Model file for the job. Use its own axes, mm. A direction names the side the tool comes from. Give positions to 0.01 mm unless a question says otherwise; leave off trailing zeros. Write each loop counter-clockwise with the first axis right and the second up, starting at its lowest first coordinate (ties: lowest second). Pieces come first, ordered by that corner, then holes.
```python
from build123d import *

# Parameters (mm, degrees)
BOSS_EXTRUDE1_DEPTH  = 82.956052622
CHAMFER1_SIZE        = 83.058
CHAMFER1_SIZE_2      = 29.329393675
BOSS_EXTRUDE3_START  = 2.592376644
BOSS_EXTRUDE3_DEPTH  = 72.586546044
CHAMFER6_SIZE        = 72.644
CHAMFER6_SIZE_2      = 25.663219438
BOSS_EXTRUDE19_DEPTH = 25.4
BOSS_EXTRUDE20_DEPTH = 25.4
BOSS_EXTRUDE21_DEPTH = 25.4
BOSS_EXTRUDE23_DEPTH = 25.4
BOSS_EXTRUDE26_START = 38.1
BOSS_EXTRUDE26_DEPTH = 12.7
BOSS_EXTRUDE27_START = -25.4
BOSS_EXTRUDE27_DEPTH = 12.7
MIRROR2_START        = 38.1
MIRROR2_COPY_2_DEPTH = 12.7
MIRROR2_START_2      = -25.4
MIRROR2_COPY_3_DEPTH = 12.7
MIRROR2_COPY_5_DEPTH = 12.7
MIRROR2_COPY_6_DEPTH = 12.7


with BuildPart() as part:
    # Sketch1 → Boss-Extrude1 (new body)
    with BuildSketch(Plane(origin=(0, 0, 0), x_dir=(1, 0, 0), z_dir=(0, 1, 0))):
        Polygon((-50.8, -29.329393675), (0, 58.65878735), (50.8, -29.329393675), align=None)
    extrude(amount=BOSS_EXTRUDE1_DEPTH)

    # Chamfer1
    # the kernel refuses this chamfer: 83.058, 29.329393675 mm, written as the material it takes off along each edge
    with BuildSketch(Plane(origin=(-158.547298904, 82.956052622, 215.953189756), x_dir=(-0.011114252752895883, -0.9999176455327007, -0.006416816818725978), z_dir=(0.5000000000000001, 0, -0.8660254037844387)), Plane(origin=(266.294597809, 82.956052622, 29.329393675), x_dir=(0, -0.9999176455327007, 0.012833633637452178), z_dir=(-1, 0, 0)), Plane(origin=(-107.747298904, 82.956052622, -245.28258343), x_dir=(0.011114252752896008, -0.9999176455327007, -0.006416816818726048), z_dir=(0.49999999999999994, 0, 0.8660254037844387))) as chamfer1_piece_1:
        Polygon((CHAMFER1_SIZE * 0.999917645533, -CHAMFER1_SIZE * 0.0128336336375), (-CHAMFER1_SIZE_2 * 0.0128336336374, -CHAMFER1_SIZE_2 * 0.999917645527), (0, 0), align=None)
    extrude(amount=532.589195618, mode=Mode.SUBTRACT)


with BuildPart() as body_2:
    # Sketch2 → Boss-Extrude3 (new body)
    with BuildSketch(Plane(origin=(0, 0, 0), x_dir=(1, 0, 0), z_dir=(0, 1, 0)).offset(BOSS_EXTRUDE3_START)):
        Polygon((-44.45, -25.663219465), (0, 51.326438931), (44.45, -25.663219465), align=None)
    extrude(amount=BOSS_EXTRUDE3_DEPTH)

    # Chamfer6
    # the kernel refuses this chamfer: 72.644, 25.663219438 mm, written as the material it takes off along each edge
    with BuildSketch(Plane(origin=(-94.237538797, 75.178922689, -214.550644108), x_dir=(0.011118590367512081, -0.9999175812357334, -0.0064193211416922824), z_dir=(0.5000000000000001, 0, 0.8660254037844386)), Plane(origin=(-138.687538797, 75.178922689, 188.887424643), x_dir=(-0.011118590367511921, -0.9999175812357334, -0.006419321141692186), z_dir=(0.49999999999999994, 0, -0.8660254037844387)), Plane(origin=(232.925077595, 75.178922689, 25.663219465), x_dir=(0, -0.9999175812357332, 0.012838642283384548), z_dir=(-1, 0, 0))) as chamfer6_piece_1:
        Polygon((CHAMFER6_SIZE * 0.999917581236, -CHAMFER6_SIZE * 0.0128386422834), (-CHAMFER6_SIZE_2 * 0.0128386422834, -CHAMFER6_SIZE_2 * 0.999917581236), (0, 0), align=None)
    extrude(amount=465.850155189, mode=Mode.SUBTRACT)

    # Sketch19 → Boss-Extrude19 (add)
    with BuildSketch(Plane(origin=(0, 8.341471254, 23.611918188), x_dir=(1, 0, 0), z_dir=(0, 0.3330989621400992, 0.9428918715426434))):
        Polygon((0, 70.885595133), (-44.414844608, -6.097300002), (44.414844608, -6.097300002), align=None)
    extrude(amount=BOSS_EXTRUDE19_DEPTH)

    # Sketch20 → Boss-Extrude20 (add)
    with BuildSketch(Plane(origin=(-20.448520983, 8.341471254, -11.805959094), x_dir=(-0.43652342739361594, 0.1780689969978707, 0.8818949651997697), z_dir=(-0.8165683137777828, 0.3330989621400992, -0.47144593577132166))):
        Polygon((13.387035379, 69.610019986), (42.464106341, -14.375505607), (-44.767106565, 2.400345516), align=None)
    extrude(amount=BOSS_EXTRUDE20_DEPTH)

    # Sketch21 → Boss-Extrude21 (add)
    with BuildSketch(Plane(origin=(20.448520983, 8.341471254, -11.805959094), x_dir=(-0.43652342739361605, -0.1780689969978708, -0.8818949651997696), z_dir=(0.8165683137777828, 0.3330989621400991, -0.47144593577132177))):
        Polygon((-13.387035361, 69.610020002), (-42.464106341, -14.375505607), (44.767106565, 2.400345516), align=None)
    extrude(amount=BOSS_EXTRUDE21_DEPTH)

    # Sketch22 → Boss-Extrude23 (add)
    with BuildSketch(Plane.XZ.offset(-2.592376644)):
        Polygon((44.414844608, 25.64292249), (-44.414844608, 25.64292249), (0, -51.285844981), align=None)
    extrude(amount=BOSS_EXTRUDE23_DEPTH)


with BuildPart() as part_1:
    add(part.part)

    # Combine3: cut body 2
    add(body_2.part, mode=Mode.SUBTRACT)

    # Sweep2: sweep along a path in Sketch25
    with BuildLine(Plane(origin=(0, 0, 0), x_dir=(0, 0, -1), z_dir=(1, 0, 0))) as sweep2_path:
        Line((-29.293394075, 0), (-41.26870121, 4.228713638))
        ThreePointArc((-41.26870121, 4.228713638), (-44.883330876, 7.477532809), (-45.141997958, 12.330724024))
    # Sketch24 → Sweep2 (sweep)
    with BuildSketch(Plane(origin=(0, 9.197233007, 26.045672391), x_dir=(1, 0, 0), z_dir=(0, 0.33296957778049097, 0.9429375696580775))):
        Polygon((-50.737646864, -9.753809057), (50.737646864, -9.753809057), (50.03399067, -8.533709325), (-50.03399067, -8.533709325), align=None)
    sweep2 = sweep(path=sweep2_path.line)

    # Sketch26 → Boss-Extrude26 (add)
    with BuildSketch(Plane(origin=(0, 0, 0), x_dir=(0, 0, -1), z_dir=(1, 0, 0)).offset(BOSS_EXTRUDE26_START)):
        with BuildLine():
            Line((-45.504344391, 10.216367205), (-45.504344391, 0))
            Line((-45.504344391, 0), (-29.293394075, 0))
            Line((-29.293394075, 0), (-41.26870121, 4.228713638))
            ThreePointArc((-41.26870121, 4.228713638), (-44.338390388, 6.549192939), (-45.504344391, 10.216367205))
        make_face()
    boss_extrude26 = extrude(amount=-BOSS_EXTRUDE26_DEPTH)

    # Sketch26<7> → Boss-Extrude27 (add)
    with BuildSketch(Plane(origin=(0, 0, 0), x_dir=(0, 0, -1), z_dir=(1, 0, 0)).offset(BOSS_EXTRUDE27_START)):
        with BuildLine():
            Line((-45.504344391, 10.216367205), (-45.504344391, 0))
            Line((-45.504344391, 0), (-29.293394075, 0))
            Line((-29.293394075, 0), (-41.26870121, 4.228713638))
            ThreePointArc((-41.26870121, 4.228713638), (-44.338390388, 6.549192939), (-45.504344391, 10.216367205))
        make_face()
    boss_extrude27 = extrude(amount=-BOSS_EXTRUDE27_DEPTH)

    # Mirror1: Sweep2, Boss-Extrude26, Boss-Extrude27 across plane
    add(sweep2.mirror(Plane(origin=(0, 0, 0), x_dir=(0.8660254037844387, 0, 0.49999999999999994), z_dir=(-0.49999999999999983, 0, 0.8660254037844387))))
    add(boss_extrude26.mirror(Plane(origin=(0, 0, 0), x_dir=(0.8660254037844387, 0, 0.49999999999999994), z_dir=(-0.49999999999999983, 0, 0.8660254037844387))))
    add(boss_extrude27.mirror(Plane(origin=(0, 0, 0), x_dir=(0.8660254037844387, 0, 0.49999999999999994), z_dir=(-0.49999999999999983, 0, 0.8660254037844387))))

    # Mirror2 copy 1: sweep along a path in Mirror2 copy 1 path
    with BuildLine(Plane(origin=(0, 0, 0), x_dir=(-0.8660254037844385, 0, 0.5), z_dir=(-0.5000000000000001, 0, -0.8660254037844388))) as mirror2_copy_1_path:
        Line((-29.293394075, 0), (-41.26870121, 4.228713638))
        ThreePointArc((-41.26870121, 4.228713638), (-44.883330876, 7.477532809), (-45.141997958, 12.330724024))
    # Mirror2 copy 1 sketch → Mirror2 copy 1 (sweep)
    with BuildSketch(Plane(origin=(22.55621395, 9.197233007, -13.022836196), x_dir=(-0.5000000000000001, 0, -0.8660254037844388), z_dir=(0.8166078895066538, 0.33296957778049074, -0.4714687848290388))):
        Polygon((-50.737646864, -9.753809057), (50.737646864, -9.753809057), (50.03399067, -8.533709325), (-50.03399067, -8.533709325), align=None)
    sweep(path=mirror2_copy_1_path.line)

    # Mirror2 copy 2 sketch → Mirror2 copy 2 (add)
    with BuildSketch(Plane(origin=(0, 0, 0), x_dir=(-0.8660254037844385, 0, 0.5), z_dir=(-0.5000000000000001, 0, -0.8660254037844388)).offset(MIRROR2_START)):
        with BuildLine():
            Line((-45.504344391, 10.216367205), (-45.504344391, 0))
            Line((-45.504344391, 0), (-29.293394075, 0))
            Line((-29.293394075, 0), (-41.26870121, 4.228713638))
            ThreePointArc((-41.26870121, 4.228713638), (-44.338390388, 6.549192939), (-45.504344391, 10.216367205))
        make_face()
    extrude(amount=-MIRROR2_COPY_2_DEPTH)

    # Mirror2 copy 3 sketch → Mirror2 copy 3 (add)
    with BuildSketch(Plane(origin=(0, 0, 0), x_dir=(-0.8660254037844385, 0, 0.5), z_dir=(-0.5000000000000001, 0, -0.8660254037844388)).offset(MIRROR2_START_2)):
        with BuildLine():
            Line((-45.504344391, 10.216367205), (-45.504344391, 0))
            Line((-45.504344391, 0), (-29.293394075, 0))
            Line((-29.293394075, 0), (-41.26870121, 4.228713638))
            ThreePointArc((-41.26870121, 4.228713638), (-44.338390388, 6.549192939), (-45.504344391, 10.216367205))
        make_face()
    extrude(amount=-MIRROR2_COPY_3_DEPTH)

    # Mirror2 copy 4: sweep along a path in Mirror2 copy 4 path
    with BuildLine(Plane(origin=(0, 0, 0), x_dir=(0.8660254037844389, 0, 0.4999999999999998), z_dir=(0.49999999999999956, 0, -0.8660254037844389))) as mirror2_copy_4_path:
        Line((-29.293394075, 0), (-41.26870121, -4.228713638))
        ThreePointArc((-41.26870121, -4.228713638), (-44.883330876, -7.477532809), (-45.141997958, -12.330724024))
    # Mirror2 copy 4 sketch → Mirror2 copy 4 (sweep)
    with BuildSketch(Plane(origin=(-22.55621395, 9.197233007, -13.022836196), x_dir=(0.49999999999999956, 0, -0.8660254037844389), z_dir=(-0.8166078895066541, 0.33296957778049086, -0.4714687848290386))):
        Polygon((-50.737646864, 9.753809057), (50.737646864, 9.753809057), (50.03399067, 8.533709325), (-50.03399067, 8.533709325), align=None)
    sweep(path=mirror2_copy_4_path.line)

    # Mirror2 copy 5 sketch → Mirror2 copy 5 (add)
    with BuildSketch(Plane(origin=(0, 0, 0), x_dir=(0.8660254037844389, 0, 0.4999999999999998), z_dir=(0.49999999999999956, 0, -0.8660254037844389)).offset(MIRROR2_START)):
        with BuildLine():
            Line((-45.504344391, -10.216367205), (-45.504344391, 0))
            Line((-45.504344391, 0), (-29.293394075, 0))
            Line((-29.293394075, 0), (-41.26870121, -4.228713638))
            ThreePointArc((-41.26870121, -4.228713638), (-44.338390388, -6.549192939), (-45.504344391, -10.216367205))
        make_face()
    extrude(amount=-MIRROR2_COPY_5_DEPTH)

    # Mirror2 copy 6 sketch → Mirror2 copy 6 (add)
    with BuildSketch(Plane(origin=(0, 0, 0), x_dir=(0.8660254037844389, 0, 0.4999999999999998), z_dir=(0.49999999999999956, 0, -0.8660254037844389)).offset(MIRROR2_START_2)):
        with BuildLine():
            Line((-45.504344391, -10.216367205), (-45.504344391, 0))
            Line((-45.504344391, 0), (-29.293394075, 0))
            Line((-29.293394075, 0), (-41.26870121, -4.228713638))
            ThreePointArc((-41.26870121, -4.228713638), (-44.338390388, -6.549192939), (-45.504344391, -10.216367205))
        make_face()
    extrude(amount=-MIRROR2_COPY_6_DEPTH)


solid = part_1.part
```
1. Slice it at A-A, the plane y = 70. Write the cut outline in (x, z), and give its area (3 significant figures).
Calculated:
outline: (-7.92, 4.58) - (-5.81, 0.91) - (-3.17, 1.83) - (-3.7, 4.58) - close; (-2.11, -5.49) - (0, -9.15) - (2.11, -5.49) - (0, -3.66) - close; (3.17, 1.83) - (5.81, 0.91) - (7.92, 4.58) - (3.7, 4.58) - close
area: 34.8 mm2
2. Slice it at D-D, the plane y = 49. Write the cut outline in (x, z), and give its area (3 significant figures).
Calculated:
outline: (-20.77, 11.99) - (-18.66, 8.33) - (-16.02, 9.25) - (-16.55, 11.99) - close; (-2.11, -20.32) - (0, -23.98) - (2.11, -20.32) - (0, -18.5) - close; (16.02, 9.25) - (18.66, 8.33) - (20.77, 11.99) - (16.55, 11.99) - close
area: 34.7 mm2
3. Which spindle directions (+Z, -Z, +X, -X, +Y, -Y) get a long thin tool onto all of the face, cutting with end or side? Do faces 4 (the flat face through (-30.625, 3.294, -16.873)), 5 (the flat face through (-47.655, 2.057, 1.816)), 6 (the flat face through (-25.4, 2, 40)), 7 (the conical face through (12.98, 7.86, -65.41)), 8 (the flat face through (-22, 41.86, 14.51)). Say none if no direction does.
Calculated:
face 4: +Y
face 5: -Z, -Y
face 6: +Z, -Y
face 7: -Z
face 8: +X, -X, +Y
4. Pin check, flat tips, straight feed: P1, Ø11, axis at y = 5, z = 38.5, coming from the +X side; P2, Ø12, axis at x = 8.5, z = -42.5, coming from the +Y side; P3, Ø1, axis at x = 17, z = -53.5, coming from the +Y side; P4, Ø3, axis at y = 7, z = 40, coming from the +X side. Stop position of each tip, or through.
Calculated:
P1: stops at x = 50.74
P2: stops at y = 3.45
P3: stops at y = 5.93
P4: passes through
5. Pull direction X, two halves, no side cores. Call faces 1 (the cylindrical face through (37.545, 7.953, -22.486)), 2 (the flat face through (0.7, 3.294, 34.959)), 3 (the conical face through (63.12, 7.87, 21.46)): +X half, -X half, draft (parallel to the pull), parting line (faces both ways), or undercut.
Calculated:
face 1: undercut
face 2: draft
face 3: +X half
6. Probe probe 1 along Z at (x, y) = (-41.5, 9); probe 2 along X at (y, z) = (6.5, -51.5); probe 3 along Y at (x, z) = (36.5, 28). List the from-to ranges inside material, lowest first.
Calculated:
probe 1: z = -18.89 to -16.4, 23.03 to 26.12, 44.14 to 45.39
probe 2: x = -22.81 to -19.56, -1.44 to 1.44, 19.56 to 22.81
probe 3: y = 0 to 3.43
7. Slice it at C-C, the plane x = -42. State how many separate pieces and enclosed holes the cut face has, and give its area (3 significant figures).
Calculated:
separate pieces: 3
enclosed holes: 0
area: 134 mm2
8. Slice it at B-B, the plane z = 34.5. Write the cut outline in (x, y), and give its area (3 significant figures).
Calculated:
outline: (-50.74, 1.84) - (-38.1, 1.84) - (-38.1, 0) - (-25.4, 0) - (-25.4, 1.84) - (25.4, 1.84) - (25.4, 0) - (38.1, 0) - (38.1, 1.84) - (50.74, 1.84) - (50.03, 3.13) - (-50.03, 3.13) - close
area: 177 mm2
